For this review, take the finished solid that the model builds, in its own axes (mm). A direction names the side the tool comes from. Coordinates: 2 decimals unless noted, no trailing zeros. Write each loop counter-clockwise with the first axis right and the second up, starting at its lowest first coordinate (ties: lowest second). Pieces come first, ordered by that corner, then holes. Notation, with made-up numbers: (75, -5.5) -> (90, -5.5) arc R21 ccw to (90, 20.5) -> close; hole circle Ø11 at (7, -10). An arc over 180 degrees is marked (long way). One line per item, written item: value. Start each with the question number.
1) For probe 1 along Z at (x, y) = (35.5, -14.5) (3 decimals); probe 2 along Z at (x, y) = (-24.5, 33.5) (3 decimals); probe 3 along Y at (x, z) = (26, 4), list the stretches that pass through material, from the lowest coordinate up. Write a range as from..to.
2) Mouldability with a two-part tool opening along X and no side actions: class faces 4 (the flat face through (2.408, 4.09, 16.754)), 5 (the flat face through (-28.7, -35, 5)), 6 (the flat face through (-35, 19, 3.375)) as released by +X, released by -X, zero draft, split by the parting line, or undercut.
3) Add section C-C (x = -32.5). State how many separate pieces and enclosed holes the cut face has, and give its area (3 significant figures).
4) Machinability: for faces 1 (the flat face through (35, -19, 6.625)), 2 (the flat face through (9.4, 35, 5)), 3 (the flat face through (0, 0, 7.25)), which of the approach directions +Z, -Z, +X, -X, +Y, -Y give a long, thin tool a straight path to every point of the face, cutting with its end or side? Answer none if there is none.
5) Add section B-B (z = 12.25). State the section outline as (x, y) points, and give its area (3 significant figures).
6) For pin 1 Ø3 at (x, y) = (35, 15.5) entering from +Z; pin 2 Ø3.5 at (y, z) = (-21, 5) entering from +X (3 decimals); pin 3 Ø1 at (x, z) = (16.5, 5.5) entering from -Y, all flat-tipped, find the tip position at first contact; note any pin that passes through.
7) Add section A-A (z = 1.5). State the section outline as (x, y) points, and give its area (3 significant figures).
from build123d import *

# Parameters (mm, degrees)
F0_W      = 76.2
F0_H      = 76.2
F1_DEPTH  = 10
F3_DEPTH  = 7
F5_DEPTH  = 7.25
F6_W      = 19.3
F6_H      = 3.25
F8_DEPTH  = 6.6
F9_COUNT  = 4
F9_ANGLE  = 270
F11_SIZE  = 0.5
F19_DEPTH = 2.375
F19_TAPER = 3


with BuildPart() as f1:
    # F0 (on Top) → F1 (new body)
    with BuildSketch(Plane.XY):
        Rectangle(F0_W, F0_H)
    extrude(amount=F1_DEPTH)

    # F2 (on face) → F3 (join)
    with BuildSketch(Plane.XY.offset(10)):
        Polygon((5, -2.8867513459), (5, 2.8867513459), (0, 5.7735026919), (-5, 2.8867513459), (-5, -2.8867513459), (0, -5.7735026919), align=None)
    extrude(amount=F3_DEPTH)

    # F4 (on face) → F5 (cut)
    with BuildSketch(Plane(origin=(0, 0, 0), x_dir=(1, 0, 0), z_dir=(0, 0, -1))):
        Polygon((5.25, -3.0310889132), (5.25, 3.0310889132), (0, 6.0621778265), (-5.25, 3.0310889132), (-5.25, -3.0310889132), (0, -6.0621778265), align=None)
    extrude(amount=-F5_DEPTH, mode=Mode.SUBTRACT)


with BuildPart() as f8:
    # F6 (on face) → F8 (new body)
    with BuildSketch(Plane.XZ.offset(38.1)):
        with Locations((-19.05, 5)):
            Rectangle(F6_W, F6_H)
    extrude(amount=-F8_DEPTH)


with BuildPart() as f8b:
    # F6 (on face) → F8, piece 2 (new body)
    with BuildSketch(Plane.XZ.offset(38.1)):
        with Locations((19.05, 5)):
            Rectangle(F6_W, F6_H)
    extrude(amount=-F8_DEPTH)


with BuildPart() as f9_1:
    # F9: instance of F8b
    add(f8b.part.rotate(Axis((0, 0, 20.068032667), (0, 0, -1)), 1 * F9_ANGLE / (F9_COUNT - 1)))


with BuildPart() as f9_2:
    # F9: instance of F8b
    add(f8b.part.rotate(Axis((0, 0, 20.068032667), (0, 0, -1)), 2 * F9_ANGLE / (F9_COUNT - 1)))


with BuildPart() as f9_3:
    # F9: instance of F8b
    add(f8b.part.rotate(Axis((0, 0, 20.068032667), (0, 0, -1)), 3 * F9_ANGLE / (F9_COUNT - 1)))


with BuildPart() as f9_4:
    # F9: instance of F8
    add(f8.part.rotate(Axis((0, 0, 20.068032667), (0, 0, -1)), 1 * F9_ANGLE / (F9_COUNT - 1)))


with BuildPart() as f9_5:
    # F9: instance of F8
    add(f8.part.rotate(Axis((0, 0, 20.068032667), (0, 0, -1)), 2 * F9_ANGLE / (F9_COUNT - 1)))


with BuildPart() as f9_6:
    # F9: instance of F8
    add(f8.part.rotate(Axis((0, 0, 20.068032667), (0, 0, -1)), 3 * F9_ANGLE / (F9_COUNT - 1)))


with BuildPart() as f1_1:
    add(f1.part)

    # F10: cut F9_3, F9_6, F9_2, F9_5, F9_1, F9_4, F8b, F8
    add(f9_3.part, mode=Mode.SUBTRACT)
    add(f9_6.part, mode=Mode.SUBTRACT)
    add(f9_2.part, mode=Mode.SUBTRACT)
    add(f9_5.part, mode=Mode.SUBTRACT)
    add(f9_1.part, mode=Mode.SUBTRACT)
    add(f9_4.part, mode=Mode.SUBTRACT)
    add(f8b.part, mode=Mode.SUBTRACT)
    add(f8.part, mode=Mode.SUBTRACT)

    # F11
    f11_edges = [f1_1.edges().sort_by_distance(p)[0] for p in [
        (5, 0, 17),
        (2.5, 4.330127, 17),
        (-2.5, 4.330127, 17),
        (-5, 0, 17),
        (-2.5, -4.330127, 17),
        (2.5, -4.330127, 17),
        (2.625, 4.546633, 0),
        (5.25, 0, 0),
        (2.625, -4.546633, 0),
        (-2.625, -4.546633, 0),
        (-5.25, 0, 0),
        (-2.625, 4.546633, 0),
        (38.1, -19.05, 6.625),
        (38.1, -9.4, 5),
        (38.1, -19.05, 3.375),
        (38.1, -28.7, 5),
        (38.1, 19.05, 3.375),
        (38.1, 9.4, 5),
        (38.1, 28.7, 5),
        (38.1, 19.05, 6.625),
        (19.05, 38.1, 6.625),
        (28.7, 38.1, 5),
        (9.4, 38.1, 5),
        (19.05, 38.1, 3.375),
        (28.7, -38.1, 5),
        (19.05, -38.1, 6.625),
        (9.4, -38.1, 5),
        (19.05, -38.1, 3.375),
        (-9.4, -38.1, 5),
        (-19.05, -38.1, 6.625),
        (-19.05, -38.1, 3.375),
        (-28.7, -38.1, 5),
        (-38.1, -28.7, 5),
        (-38.1, -19.05, 6.625),
        (-38.1, -9.4, 5),
        (-38.1, -19.05, 3.375),
        (-38.1, 9.4, 5),
        (-38.1, 19.05, 6.625),
        (-38.1, 28.7, 5),
        (-38.1, 19.05, 3.375),
        (-19.05, 38.1, 6.625),
        (-28.7, 38.1, 5),
        (-9.4, 38.1, 5),
        (-19.05, 38.1, 3.375),
    ]]
    chamfer(f11_edges, length=F11_SIZE)

    # F18 (on face) → F19 (cut)
    with BuildSketch(Plane.XY.offset(10)):
        Polygon((-29.2, 35.1), (-35.1, 29.2), (-35.1, -29.2), (-29.2, -35.1), (29.2, -35.1), (35.1, -29.2), (35.1, 29.2), (29.2, 35.1), align=None)
        Polygon((0, -8.0829037687), (-7, -4.0414518843), (-7, 4.0414518843), (0, 8.0829037687), (7, 4.0414518843), (7, -4.0414518843), align=None, mode=Mode.SUBTRACT)
    extrude(amount=-F19_DEPTH, taper=F19_TAPER, mode=Mode.SUBTRACT)


solid = f1_1.part
Numbers:
1. probe 1: 0..3.375, 6.625..10
1. probe 2: 0..3.375, 6.625..7.625
1. probe 3: -31.5..31.5
2. face 4: released by +X
2. face 5: undercut
2. face 6: zero draft
3. separate pieces: 1
3. enclosed holes: 2
3. area: 486 mm²
4. face 1: +X
4. face 2: +Y
4. face 3: -Z
5. outline: (-5, -2.89) -> (0, -5.77) -> (5, -2.89) -> (5, 2.89) -> (0, 5.77) -> (-5, 2.89) -> close
5. area: 86.6 mm²
6. pin 1: z = 10
6. pin 2: x = 37.725
6. pin 3: y = -31.5
7. outline: (-38.1, -38.1) -> (38.1, -38.1) -> (38.1, 38.1) -> (-38.1, 38.1) -> close; hole (-5.25, -3.03) -> (0, -6.06) -> (5.25, -3.03) -> (5.25, 3.03) -> (0, 6.06) -> (-5.25, 3.03) -> close
7. area: 5,710 mm²
